Check sheet for the modelled part. Datum: model origin and axes. Units: mm. A direction names the side the tool comes from. Coordinates: 2 decimals unless noted, no trailing zeros. Write each loop counter-clockwise with the first axis right and the second up, starting at its lowest first coordinate (ties: lowest second). Pieces come first, ordered by that corner, then holes. Notation, with made-up numbers: M 36,-18 L 72,-18 A32 ccw 72,8 Z; hole C 51.5,-2.75 d9. An arc over 180 degrees is marked long. Answer as CSV lines item,"result". Start each with the question number.
Q1. Sectioned sample at A-A, the plane z = 27.5. Record the cut outline in (x, y).
Q2. Sectioned sample at B-B, the plane y = -30. Record the cut outline in (x, z), then the cut area to 3 significant figures.
Q3. Sectioned sample at C-C, the plane x = -20.5. Record the cut outline in (y, z), then the cut area to 3 significant figures.
Q4. Access from +Z, -Z, +X, -X, +Y, -Y to the whole of each face (thin tool, end or side, straight path). Record for faces 1 (the flat face through (-10, -19, 0)), 2 (the flat face through (-10, -23, 6.35)), 3 (the flat face through (-27, -12.177, 21)).
Q5. Thickness scan on line 1 along Y through (x, z) = (-31, 13); line 2 along Z through (x, y) = (-42, -27); line 3 along Y through (x, z) = (19.5, 6). Record the ranges inside material, lowest first. Write a range as from..to.
Q6. Mould release check, pull along Y, two halves, no side actions. Record for faces 4 (the cylindrical face through (-12.65, -6.17, 16.74)), 5 (the cylindrical face through (13.76, -8.61, 3.22)), 6 (the flat face through (-10, -38.1, 3)): pulls with the +Y half, pulls with the -Y half, needs draft (parallel to the pull), parting line crosses it, or undercut.
Q7. Sectioned sample at D-D, the plane z = 37. Record the cut outline in (x, y), then the cut area to 3 significant figures.
Q8. Depth check by flat-ended pin: pin 1 Ø10 at (x, y) = (-24, -24) entering from +Z; pin 2 Ø12 at (y, z) = (-4.5, 19) entering from +X; pin 3 Ø1 at (x, y) = (-5, -24) entering from +Z. Enter the tip coordinate at first touch or a pass-through.
from build123d import *

# Parameters (mm, degrees)
F0_W      = 69.85
F0_H      = 44.45
F1_DEPTH  = 38.1
F3_DEPTH  = 44.451
F5_DEPTH  = 31.75
F6_DEPTH  = 5.08
F7_DEPTH  = 6.35
F8_DEPTH  = 5.08
F10_DEPTH = 12.1779236892
F11_R     = 7.0905060621
F12_DEPTH = 25.9240763108
F13_DEPTH = 38.102
F14_R     = 3.5131163542
F14_R_2   = 3.5285454021
F14_R_3   = 3.4395422414
F15_DEPTH = 6.351


with BuildPart() as f1:
    # F0 (on Front) → F1 (new body)
    with BuildSketch(Plane.XZ):
        with Locations((-9.9012593745, 22.225)):
            Rectangle(F0_W, F0_H)
    extrude(amount=F1_DEPTH)

    # F2 (on face) → F3 (cut, through all)
    with BuildSketch(Plane.XY.offset(44.45)):
        with BuildLine():
            ThreePointArc((-38.0205141645, -38.1), (-42.7526228642, -35.9796762697), (-44.8262593745, -31.2269236892))
            Line((-44.8262593745, -31.2269236892), (-44.8262593745, -38.1))
            Line((-44.8262593745, -38.1), (-38.0205141645, -38.1))
        make_face()
        with BuildLine():
            ThreePointArc((25.0237406255, -32.3781482875), (22.8273562196, -36.1989998927), (18.8512764871, -38.1))
            Line((18.8512764871, -38.1), (25.0237406255, -38.1))
            Line((25.0237406255, -38.1), (25.0237406255, -32.3781482875))
        make_face()
    extrude(amount=-F3_DEPTH, mode=Mode.SUBTRACT)

    # F4 (on face) → F5 (cut)
    with BuildSketch(Plane.XY.offset(44.45)):
        with BuildLine():
            Line((-0.3762593745, -12.1769236892), (-44.8262593745, -12.1769236892))
            Line((-44.8262593745, -12.1769236892), (-44.8262593745, -31.2269236892))
            ThreePointArc((-44.8262593745, -31.2269236892), (-42.7526228642, -35.9796762697), (-38.0205141645, -38.1))
            Line((-38.0205141645, -38.1), (18.8512764871, -38.1))
            ThreePointArc((18.8512764871, -38.1), (22.8273562196, -36.1989998927), (25.0237406255, -32.3781482875))
            Line((25.0237406255, -32.3781482875), (25.0237406255, 0))
            Line((25.0237406255, 0), (-0.3762593745, 0))
            Line((-0.3762593745, 0), (-0.3762593745, -12.1769236892))
        make_face()
    extrude(amount=-F5_DEPTH, mode=Mode.SUBTRACT)

    # F6 (add): a face of the model
    f6_faces = [f1.faces().sort_by_distance(p)[0] for p in [
        (-6.6136162869, -22.2162080718, 12.7),
    ]]
    extrude(f6_faces, amount=F6_DEPTH)

    # F7 (cut): a face of the model
    f7_faces = [f1.faces().sort_by_distance(p)[0] for p in [
        (-6.6136162869, -22.2162080718, 17.78),
    ]]
    extrude(f7_faces, amount=-F7_DEPTH, mode=Mode.SUBTRACT)

    # F8 (cut): a face of the model
    f8_faces = [f1.faces().sort_by_distance(p)[0] for p in [
        (-6.6136162869, -22.2162080718, 11.43),
    ]]
    extrude(f8_faces, amount=-F8_DEPTH, mode=Mode.SUBTRACT)

    # F9 (on face) → F10 (cut, through all)
    with BuildSketch(Plane.XZ.offset(12.1769236892)):
        with BuildLine():
            ThreePointArc((-44.8262593745, 35.5440117419), (-42.2872783605, 41.3383758962), (-36.7792046519, 44.45))
            Line((-36.7792046519, 44.45), (-44.8262593745, 44.45))
            Line((-44.8262593745, 44.45), (-44.8262593745, 35.5440117419))
        make_face()
        with BuildLine():
            Line((-0.3762593745, 44.45), (-31.7305137767, 44.45))
            ThreePointArc((-31.7305137767, 44.45), (-22.5706200379, 40.403916894), (-18.5634717345, 31.2269236892))
            ThreePointArc((-18.5634717345, 31.2269236892), (-12.5199705056, 16.5585677002), (-0.3762593745, 6.35))
            Line((-0.3762593745, 6.35), (-0.3762593745, 44.45))
        make_face()
    extrude(amount=-F10_DEPTH, mode=Mode.SUBTRACT)

    # F11 (on face) → F12 (join, through all)
    with BuildSketch(Plane.XZ.offset(12.1769236892)):
        with Locations((-32.3421357847, 30.6738090409)):
            Circle(F11_R)
    extrude(amount=F12_DEPTH)

    # F13 (cut, through all): a face of the model
    f13_faces = [f1.faces().sort_by_distance(p)[0] for p in [
        (-32.3421357847, -38.101, 30.6738090409),
    ]]
    extrude(f13_faces, amount=-F13_DEPTH, mode=Mode.SUBTRACT)

    # F14 (on face) → F15 (cut, through all)
    with BuildSketch(Plane.XY.offset(6.35)):
        with Locations((16.5488310158, -6.4756297506)):
            Circle(F14_R)
        with Locations((17.7833885895, -30.7578051752)):
            Circle(F14_R_2)
        with Locations((-37.6456809362, -30.9227637617)):
            Circle(F14_R_3)
    extrude(amount=-F15_DEPTH, mode=Mode.SUBTRACT)


solid = f1.part
Output:
1,outline,"M -44.83,-12.18 L -38.68,-12.18 L -38.68,0 L -44.83,0 Z; M -26,-12.18 L -17.78,-12.18 L -17.78,0 L -26,0 Z"
2,outline,"M -44.83,0 L -40.96,0 L -40.96,6.35 L -44.83,6.35 Z; M -34.33,0 L 14.34,0 L 14.34,6.35 L -34.33,6.35 Z; M 21.23,0 L 25.02,0 L 25.02,6.35 L 21.23,6.35 Z"
2,area,"358 mm^2"
3,outline,"M -38.1,0 L 0,0 L 0,37.74 L -12.18,37.74 L -12.18,6.35 L -38.1,6.35 Z"
3,area,"624 mm^2"
4,face 1,"-Z, +X, -X, +Y, -Y"
4,face 2,"+Z, +X, -Y"
4,face 3,"+Z, +X, -X, -Y"
5,line 1,"y = -12.18..0"
5,line 2,"z = 0..6.35"
5,line 3,"y = -37.98..-33.84, -27.67..-8.38, -4.57..0"
6,face 4,"needs draft"
6,face 5,"undercut"
6,face 6,"pulls with the -Y half"
7,outline,"M -44.58,-12.18 L -35.54,-12.18 L -35.54,0 L -44.58,0 Z; M -29.14,-12.18 L -20.09,-12.18 L -20.09,0 L -29.14,0 Z"
7,area,"220 mm^2"
8,pin 1,"stops at z = 6.35"
8,pin 2,"stops at x = -9.51"
8,pin 3,"stops at z = 6.35"
